The drawing under review shows one solid part. Ordinate dimensions are in mm from its lowest x, y, z. Round coordinates to 2 decimals unless told otherwise and drop trailing zeros. Write each loop counter-clockwise with the first axis right and the second up, starting at its lowest first coordinate (ties: lowest second). Pieces come first, ordered by that corner, then holes. Notation, with made-up numbers: (2.25, 46) -> (46.25, 46) arc R12 cw to (46.25, 51) -> close; hole circle Ø2 at (-6.5, 83.25). An arc over 180 degrees is marked (long way). Write item = value, one per line. Start each with the question number.
Item 1: Add section D-D, the plane x = 11. State the section outline as (y, z) points.
Item 2: Add section A-A, the plane z = 11. State the section outline as (x, y) points, then the cut area to 3 significant figures.
Item 3: Mouldability with a two-part tool opening along Y and no side actions: class the marked faces 1 and 2 as released by +Y, released by -Y, zero draft, split by the parting line, or undercut.
Item 4: For pin 1 Ø1 at (x, y) = (23, 1) entering from -Z; pin 2 Ø2 at (x, y) = (9, 1) entering from -Z; pin 3 Ø1.2 at (x, y) = (5.5, 2) entering from +Z, all flat-tipped, find the tip position at first contact; note any pin that passes through.
Item 5: To check wall thickness, follow L1, parallel to X at y = 0.3, z = 13.5; L2, parallel to Z at x = 38.5, y = 3.5; L3, parallel to X at y = 2.4, z = 6.5. State the ranges of each line that lie inside material, in increasing order.
Item 6: Add section B-B, the plane y = 3.2. State the section outline as (x, z) points, then the cut area to 3 significant figures.
Item 7: Add section C-C, the plane x = 5. State the section outline as (y, z) points.
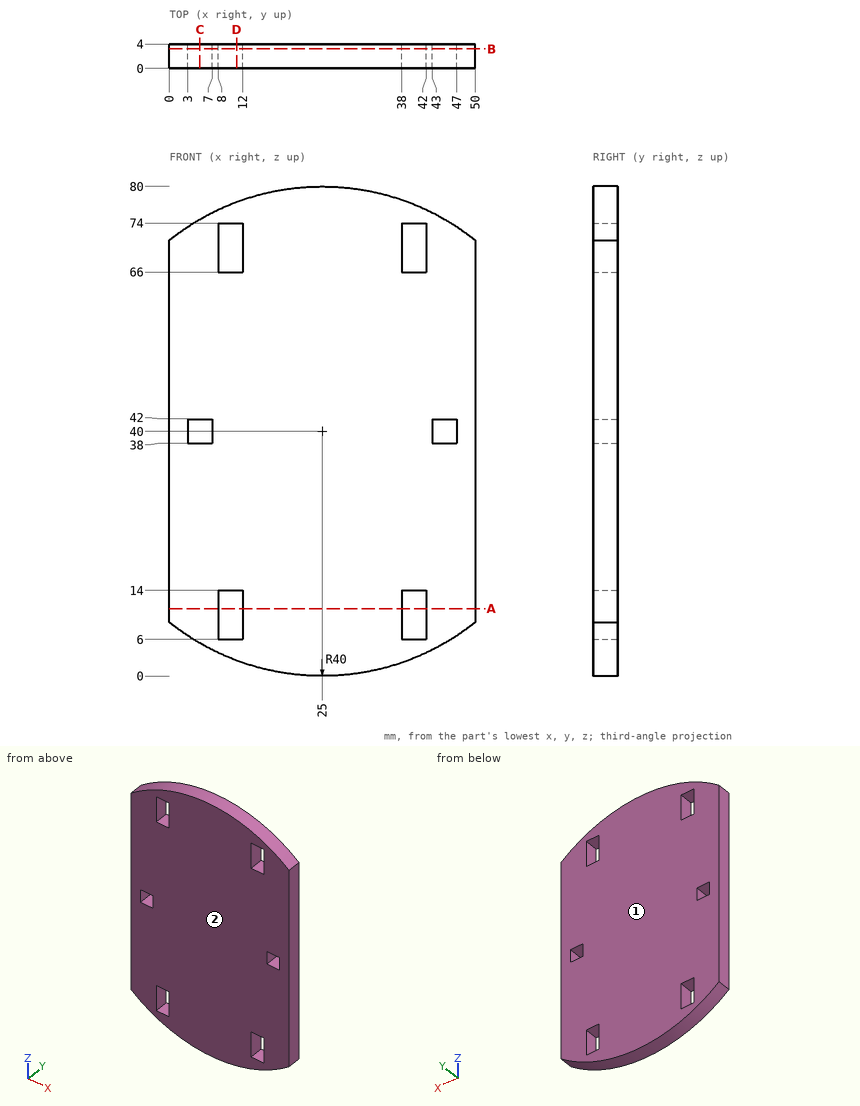
Result set:
q1.outline = (0, 2.53) -> (4, 2.53) -> (4, 6) -> (0, 6) -> close; (0, 14) -> (4, 14) -> (4, 66) -> (0, 66) -> close; (0, 74) -> (4, 74) -> (4, 77.47) -> (0, 77.47) -> close
q2.outline = (0, 0) -> (8, 0) -> (8, 4) -> (0, 4) -> close; (12, 0) -> (38, 0) -> (38, 4) -> (12, 4) -> close; (42, 0) -> (50, 0) -> (50, 4) -> (42, 4) -> close
q2.area = 168 mm²
q3.face_1 = released by +Y
q3.face_2 = released by -Y
q4.pin_1 = 0.03
q4.pin_2 = 2.92
q4.pin_3 = 75.25
q5.L1 = 0 to 8, 12 to 38, 42 to 50
q5.L2 = 2.35 to 6, 14 to 66, 74 to 77.65
q5.L3 = 3.14 to 8, 12 to 38, 42 to 46.86
q6.outline = (0, 8.78) arc R40 ccw to (50, 8.78) -> (50, 71.22) arc R40 ccw to (0, 71.22) -> close; hole (3, 38) -> (7, 38) -> (7, 42) -> (3, 42) -> close; hole (8, 6) -> (12, 6) -> (12, 14) -> (8, 14) -> close; hole (8, 66) -> (12, 66) -> (12, 74) -> (8, 74) -> close; hole (38, 6) -> (42, 6) -> (42, 14) -> (38, 14) -> close; hole (38, 66) -> (42, 66) -> (42, 74) -> (38, 74) -> close; hole (43, 38) -> (47, 38) -> (47, 42) -> (43, 42) -> close
q6.area = 3,560 mm²
q7.outline = (0, 5.36) -> (4, 5.36) -> (4, 38) -> (0, 38) -> close; (0, 42) -> (4, 42) -> (4, 74.64) -> (0, 74.64) -> close
